```python
from build123d import *

# Parameters (mm, degrees)
BOSS_EXTRUDE1_DEPTH = 88.9
SKETCH2_R           = 3.175
SKETCH2_R_2         = 1.27
SKETCH2_W           = 12.784255415
SKETCH2_H           = 12.760259732
CUT_EXTRUDE1_DEPTH  = 81.28


with BuildPart() as part:
    # Sketch1 → Boss-Extrude1 (new body)
    with BuildSketch(Plane(origin=(0, 0, 0), x_dir=(0, 0, -1), z_dir=(1, 0, 0))):
        Polygon((6.35, 11.43), (6.35, -71.755), (0, -71.755), (0, 11.43), (0, 43.18), (-15.875, 43.18), (-15.875, 71.755), (15.875, 71.755), (15.875, 8.255), (9.525, 8.255), (9.525, 65.405), (-9.525, 65.405), (-9.525, 49.53), (6.35, 49.53), align=None)
    extrude(amount=BOSS_EXTRUDE1_DEPTH)

    # Sketch2 → Cut-Extrude1 (cut)
    with BuildSketch(Plane(origin=(0, 0, -15.875), x_dir=(-1, 0, 0), z_dir=(0, 0, -1))):
        with Locations(Location((-44.45, 27.305, 0), (0, 0, 90))):
            Circle(SKETCH2_R)
        with Locations(Location((-80.01, 27.305, 0), (0, 0, 90))):
            Circle(SKETCH2_R)
        with Locations(Location((-80.01, 14.605, 0), (0, 0, 90))):
            Circle(SKETCH2_R)
        with Locations(Location((-44.45, 14.605, 0), (0, 0, 90))):
            Circle(SKETCH2_R)
        with Locations(Location((-8.89, 14.605, 0), (0, 0, 90))):
            Circle(SKETCH2_R)
        with Locations(Location((-8.89, 27.305, 0), (0, 0, 90))):
            Circle(SKETCH2_R)
        with Locations(Location((-77.47, -18.415, 0), (0, 0, 90))):
            Circle(SKETCH2_R_2)
        with Locations(Location((-77.47, -36.195, 0), (0, 0, 90))):
            Circle(SKETCH2_R_2)
        with Locations(Location((-77.47, -53.975, 0), (0, 0, 90))):
            Circle(SKETCH2_R_2)
        with Locations(Location((-11.43, -53.975, 0), (0, 0, 90))):
            Circle(SKETCH2_R_2)
        with Locations(Location((-11.43, -36.195, 0), (0, 0, 90))):
            Circle(SKETCH2_R_2)
        with Locations(Location((-11.43, -18.415, 0), (0, 0, 90))):
            Circle(SKETCH2_R_2)
        with Locations((-73.617872293, -6.922794841)):
            Rectangle(SKETCH2_W, SKETCH2_H)
    extrude(amount=-CUT_EXTRUDE1_DEPTH, mode=Mode.SUBTRACT)


solid = part.part
```
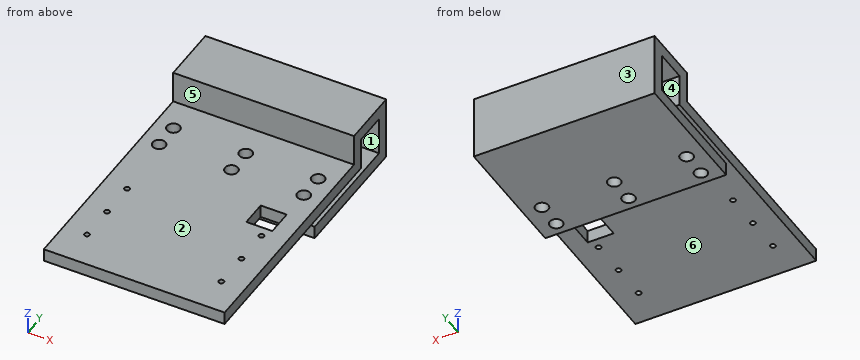
CAD build for the part. Positions are in the model's coordinates, mm. Face numbers are marked on the shaded views. A direction names the side the tool comes from. Round coordinates to 2 decimals unless told otherwise and drop trailing zeros. Order: outer loops, then holes, each group sorted by start corner. A loop starts at its lowest first (then second) coordinate and runs counter-clockwise, first axis right, second up. Notation, with made-up numbers: (31, 30.5) -> (47, 30.5) arc R27 ccw to (47, 64.5) -> close; hole circle Ø5 at (83, 82.25). An arc over 180 degrees is marked (long way). One line per question, with ' | ' between items.
Q1. Two-plate mould, pull along Z, no slides. Class the marked faces 1, 2 and 3: released by +Z, released by -Z, zero draft, split by the parting line, or undercut.
Completed:
face 1: undercut | face 2: released by +Z | face 3: zero draft
Q2. Which spindle directions (+Z, -Z, +X, -X, +Y, -Y) get a long thin tool onto all of the face, cutting with end or side? Do the marked faces 4, 5 and 6. Say none if no direction does.
Completed:
face 4: +X, -X | face 5: +Z, +X, -X, -Y | face 6: +X, -X, -Y
Q3. Slice it at B-B (z = -1.5). Give the number of separate pieces and of enclosed holes in the cut face, then the cut area to 3 significant figures.
Completed:
separate pieces: 2 | enclosed holes: 13 | area: 11,000 mm^2
Q4. Slice it at C-C (y = 53.5). Write the cut outline in (x, z) (3 decimals), then the cut area to 3 significant figures.
Completed:
outline: (0, -15.875) -> (88.9, -15.875) -> (88.9, -9.525) -> (0, -9.525) -> close; (0, 9.525) -> (88.9, 9.525) -> (88.9, 15.875) -> (0, 15.875) -> close | area: 1,130 mm^2
Q5. Drop flat-ended pins along their axis: pin 1 (1.5 mm diameter, centred on x = 77.47, y = -53.975, fed in from +Z); pin 2 (4 mm diameter, centred on x = 77.47, y = -36.195, fed in from -Z); pin 3 (8 mm diameter, centred on x = 32.5, z = 5.5, fed in from -Y); pin 4 (3 mm diameter, centred on x = 11.43, y = -53.975, fed in from +Z). Give the stop position or say it passes through.
Completed:
pin 1: passes through | pin 2: stops at z = -6.35 | pin 3: stops at y = 43.18 | pin 4: stops at z = 0
Q6. Slice it at A-A (x = 44.45). Write the cut outline in (y, z) (3 decimals).
Completed:
outline: (-71.755, -6.35) -> (11.43, -6.35) -> (11.43, 0) -> (-71.755, 0) -> close; (8.255, -15.875) -> (11.43, -15.875) -> (11.43, -9.525) -> (8.255, -9.525) -> close; (17.78, -15.875) -> (24.13, -15.875) -> (24.13, -9.525) -> (17.78, -9.525) -> close; (17.78, -6.35) -> (24.13, -6.35) -> (24.13, 0) -> (17.78, 0) -> close; (30.48, -15.875) -> (71.755, -15.875) -> (71.755, 15.875) -> (43.18, 15.875) -> (43.18, 0) -> (30.48, 0) -> (30.48, -6.35) -> (49.53, -6.35) -> (49.53, 9.525) -> (65.405, 9.525) -> (65.405, -9.525) -> (30.48, -9.525) -> close
Q7. Slice it at D-D (x = 19). Write the cut outline in (y, z) (3 decimals).
Completed:
outline: (-71.755, -6.35) -> (49.53, -6.35) -> (49.53, 9.525) -> (65.405, 9.525) -> (65.405, -9.525) -> (8.255, -9.525) -> (8.255, -15.875) -> (71.755, -15.875) -> (71.755, 15.875) -> (43.18, 15.875) -> (43.18, 0) -> (-71.755, 0) -> close
Q8. Probe probe 1 along Y at (x, z) = (80, -13) (3 decimals); probe 2 along Y at (x, z) = (78.5, 3.5) (3 decimals); probe 3 along Y at (x, z) = (56.5, -5.5) (3 decimals). List the from-to ranges inside material, lowest first.
Completed:
probe 1: y = 8.255 to 11.43, 17.78 to 24.13, 30.48 to 71.755 | probe 2: y = 43.18 to 49.53, 65.405 to 71.755 | probe 3: y = -71.755 to 49.53, 65.405 to 71.755
